Check sheet for the modelled part. Datum: model origin and axes. Units: mm. Face numbers are marked on the shaded views. A direction names the side the tool comes from. Give positions to 0.01 mm unless a question says otherwise; leave off trailing zeros. Order: outer loops, then holes, each group sorted by start corner. A loop starts at its lowest first (then second) coordinate and runs counter-clockwise, first axis right, second up. Notation, with made-up numbers: M 72,66.25 L 82,66.25 A19 cw 82,88.25 Z; hole C -3.5,71 d1. An arc over 180 degrees is marked long. One line per question, with ' | ' between items. Start each with the question number.
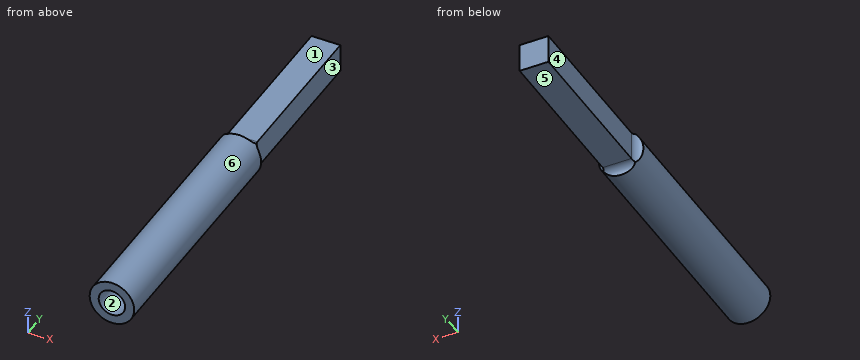
Autodesk Inventor part; units mm, degrees
ref_plane "YZ Plane" through (0, 0, 0) normal (1, 0, 0) x (0, 1, 0)
ref_plane "XZ Plane" through (0, 0, 0) normal (0, 1, 0) x (-1, 0, 0)
ref_plane "XY Plane" through (0, 0, 0) normal (0, 0, 1) x (1, 0, 0)
sketch "Sketch1" plane through (0, 0, 0) normal (0, 1, 0) x (-1, 0, 0)
  circle A0 centre (0, 0) radius 2.032
  dimension "d0" = 4.064
extrude "Extrusion1" add sketch "Sketch1" along normal blind 22.225
sketch "Sketch2" plane through (0, 22.225, 0) normal (0, 1, 0) x (1, 0, 0)
  line L0 (-1.3117, -1.3117) -> (1.3117, -1.3117)
  line L1 (1.3117, -1.3117) -> (1.3117, 1.3117)
  line L2 (1.3117, 1.3117) -> (-1.3117, 1.3117)
  line L3 (-1.3117, 1.3117) -> (-1.3117, -1.3117)
  point P0 (0, 0)
  point P1 (-1.3117, 0)
  point P2 (0, -1.3117)
  dimension "d3" = 2.6234
  dimension "d4" = 2.6234
extrude "Extrusion2" add sketch "Sketch2" along normal blind 15.24
sketch "Sketch3" plane through (0, 0, 0) normal (0, -1, 0) x (1, 0, 0)
  point P0 (0, 0)
  point P1 (0, 0)
hole "Hole1" at (0, 0, 0) direction (0, 1, 0) diameter 2.413 depth 20.32
fillet "Fillet1" radius 0.7112 4 edges at (0, 22.225, 1.3117) (1.3117, 22.225, 0) (0, 22.225, -1.3117) (-1.3117, 22.225, 0)
equation "\"d4\" = d3"
properties part number "shaft_adapter_v2" material "ABS Plastic"
Item 1: Scan lines: probe 1 along X at (y, z) = (11, 0); probe 2 along Y at (x, z) = (0, 0.6) (3 decimals). Record each from-to range of solid material in increasing order. Write a range as [from, to].
Item 2: Draft check along X on the marked faces 1, 2, 3 and 4. Enter one of: released by +X, released by -X, zero draft, split by the parting line, or undercut.
Item 3: Section check A-A, the plane z = -0.75. Record the cut outline in (x, y) (3 decimals).
Item 4: Set-up check for the marked faces 5 and 6: record each of +Z, -Z, +X, -X, +Y, -Y from which the full face is reachable in a straight line by a thin tool's end or side.
Item 5: Section check C-C, the plane y = 13.5. Record the cut outline in (x, z), then the cut area to 3 significant figures.
Item 6: Section check B-B, the plane x = 0.85. Record the cut outline in (y, z) (3 decimals).
Item 7: Go/stop test with flat-tipped pins: P1, Ø0.8, axis at y = 30.5, z = -0.5, coming from the +X side; P2, Ø1.2, axis at x = 0.5, z = 0, coming from the -Y side; P3, Ø2, axis at x = -0.5, y = 30, coming from the +Z side. Record where each tip stops, or that it passes through.
Reported:
1) probe 1: x = [-2.03, -1.21], [1.21, 2.03] | probe 2: y = [20.32, 37.465]
2) face 1: zero draft | face 2: undercut | face 3: released by +X | face 4: released by -X
3) outline: M -1.889,0 L -0.945,0 L -0.945,20.32 L 0.945,20.32 L 0.945,0 L 1.889,0 L 1.889,22.238 A0.711 cw 1.312,22.936 L 1.312,37.465 L -1.312,37.465 L -1.312,22.936 A0.711 cw -1.889,22.238 Z
4) face 5: -Z, +X, -X, +Y | face 6: +Y, -Y
5) outline: C 0,0 d4.06; hole C 0,0 d2.41 | area: 8.40 mm^2
6) outline: M 0,-1.846 L 22.247,-1.846 A0.711 cw 22.936,-1.312 L 37.465,-1.312 L 37.465,1.312 L 22.936,1.312 A0.711 cw 22.247,1.846 L 0,1.846 L 0,0.856 L 20.32,0.856 L 20.32,-0.856 L 0,-0.856 Z
7) P1: stops at x = 1.31 | P2: stops at y = 20.32 | P3: stops at z = 1.31
